from build123d import *

# Parameters (mm, degrees)
DODANIE_WYCI_GNI_CIE1_DEPTH = 220
SZKIC4_W                    = 30
SZKIC4_H                    = 23
DODANIE_WYCI_GNI_CIE3_DEPTH = 5
SZKIC5_W                    = 10
SZKIC5_H                    = 10
SZKIC5_W_2                  = 25
SZKIC5_H_2                  = 25
WYTNIJ_WYCI_GNI_CIE1_DEPTH  = 25


with BuildPart() as part:
    # Szkic1 → Dodanie-wyciągnięcie1 (new body)
    with BuildSketch(Plane.XY):
        Polygon((-22.5, -10), (52.5, -10), (52.5, -5), (22.5, -5), (22.5, 18), (17.5, 18), (17.5, 0), (-17.5, 0), (-17.5, 18), (-22.5, 18), align=None)
    extrude(amount=-DODANIE_WYCI_GNI_CIE1_DEPTH)

    # Szkic4 → Dodanie-wyciągnięcie3 (add)
    with BuildSketch(Plane.XY):
        with Locations((37.5, 6.5)):
            Rectangle(SZKIC4_W, SZKIC4_H)
    extrude(amount=-DODANIE_WYCI_GNI_CIE3_DEPTH)

    # Szkic5 → Wytnij-wyciągnięcie1 (cut)
    with BuildSketch(Plane(origin=(0, 0, 0), x_dir=(1, 0, 0), z_dir=(0, 1, 0))):
        with Locations((0, 50)):
            Rectangle(SZKIC5_W, SZKIC5_H)
        with Locations((0, 100)):
            Rectangle(SZKIC5_W, SZKIC5_H)
        with Locations((0, 137.5)):
            Rectangle(SZKIC5_W_2, SZKIC5_H_2)
    extrude(amount=-WYTNIJ_WYCI_GNI_CIE1_DEPTH, mode=Mode.SUBTRACT)


solid = part.part
Read the model definition and answer for the solid it produces. Units are mm, in the model's axes. A direction names the side the tool comes from. Coordinates: 2 decimals unless noted, no trailing zeros. Loops run counter-clockwise (first coordinate to the right, second up) from the corner with the lowest first, then second, coordinate; pieces in that order, holes last.
Q1. The part is cut by section D-D on z = -132. Write down the section's boundary in (x, y), and give its area (3 significant figures).
Q2. The part is cut by section C-C on x = 8. Write down the section's boundary in (y, z), and give its area (3 significant figures).
Q3. The part is cut by section A-A on x = -1. Write down the section's boundary in (y, z).
Q4. The part is cut by section B-B on y = 6.5. Write down the section's boundary in (x, z), and give its area (3 significant figures).
Q5. The mould has two halves that part along Z. Classify faces 1 (the face through (23, 1, 0)), 2 (the face through (-12.5, -5, -137)), 3 (the face through (17.5, 9, -108)): +Z half, -Z half, draft (parallel to the pull), parting line (faces both ways), or undercut.
Q6. Which of the six approach directions +Z, -Z, +X, -X, +Y, -Y give full straight-line access (tool end or side, diameter ignored) to faces 4 (the face through (22.5, 6, -111)), 5 (the face through (0, -5, -55)), 6 (the face through (0, 0, -108))?
Q7. Consider probe 1 along Z at (x, y) = (-1, -7.75); probe 2 along X at (y, z) = (9.75, -61.5); probe 3 along Z at (x, y) = (-5.5, -0.75). Determine where each line is inside the solid, lowest interval first.
Q8. Each of these flat-tipped pins is pushed along its axis until it touches: pin 1 Ø11.5 at (y, z) = (12, -110) entering from +X; pin 2 Ø15 at (x, z) = (39, -152) entering from +Y; pin 3 Ø12 at (x, y) = (34, 5.5) entering from -Z. Where does it stop, or does it pass through?
Results below:
1. outline: (-22.5, -10) - (-12.5, -10) - (-12.5, 0) - (-17.5, 0) - (-17.5, 18) - (-22.5, 18) - close; (12.5, -10) - (52.5, -10) - (52.5, -5) - (22.5, -5) - (22.5, 18) - (17.5, 18) - (17.5, 0) - (12.5, 0) - close
1. area: 530 mm2
2. outline: (-10, -220) - (0, -220) - (0, -150) - (-10, -150) - close; (-10, -125) - (0, -125) - (0, 0) - (-10, 0) - close
2. area: 1,950 mm2
3. outline: (-10, -220) - (0, -220) - (0, -150) - (-10, -150) - close; (-10, -125) - (0, -125) - (0, -105) - (-10, -105) - close; (-10, -95) - (0, -95) - (0, -55) - (-10, -55) - close; (-10, -45) - (0, -45) - (0, 0) - (-10, 0) - close
4. outline: (-22.5, -220) - (-17.5, -220) - (-17.5, 0) - (-22.5, 0) - close; (17.5, -220) - (22.5, -220) - (22.5, -5) - (52.5, -5) - (52.5, 0) - (17.5, 0) - close
4. area: 2,350 mm2
5. face 1: +Z half
5. face 2: undercut
5. face 3: draft
6. face 4: -Z, +X, +Y
6. face 5: +Y, -Y
6. face 6: +Z, -Z, +Y
7. probe 1: z = -220 to -150, -125 to -105, -95 to -55, -45 to 0
7. probe 2: x = -22.5 to -17.5, 17.5 to 22.5
7. probe 3: z = -220 to -150, -125 to 0
8. pin 1: stops at x = 22.5
8. pin 2: stops at y = -5
8. pin 3: stops at z = -5
